from build123d import *

# Parameters (mm, degrees)
PAD_DEPTH = 27


with BuildPart() as part:
    # Sketch → Pad (new body)
    with BuildSketch(Plane.YZ):
        Polygon((0, 0), (0, 1), (3, 1), (3, 6), (5, 6), (5, 2), (7, 0), align=None)
    pad = extrude(amount=PAD_DEPTH)

    # Mirrored: Pad across Sketch V_Axis
    add(pad.mirror(Plane(origin=(0, 0, 0), x_dir=(1, 0, 0), z_dir=(0, 1, 0))))


solid = part.part
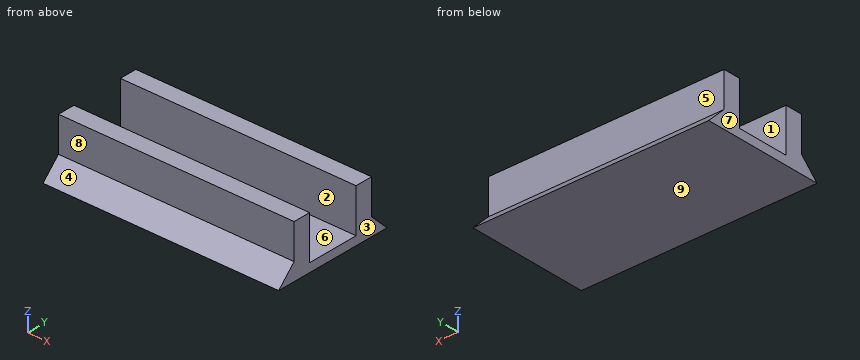
Input: part model. Units: mm. Frame: model coordinates. Face numbers are marked on the shaded views. A direction names the side the tool comes from. Give positions to 0.01 mm unless a question says otherwise; leave off trailing zeros. Loops run counter-clockwise (first coordinate to the right, second up) from the corner with the lowest first, then second, coordinate; pieces in that order, holes last. Notation, with made-up numbers: M 4.25,-33 L 16.25,-33 A10 ccw 16.25,-17 Z; hole C 1.25,61 d1. An arc over 180 degrees is marked long. Use one line per item in the form item = value.
1. Section query B-B, the plane x = 20.5. Return the cut outline in (y, z), and give its area (3 significant figures).
Numbers:
outline = M -7,0 L 7,0 L 5,2 L 5,6 L 3,6 L 3,1 L -3,1 L -3,6 L -5,6 L -5,2 Z
area = 34.0 mm²
2. Line query: L1, parallel to Y at x = 22.75, z = 3.4; L2, parallel to Z at x = 1.75, y = 1; L3, parallel to Y at x = 6.25, z = 1.4. Output: solid intervals per line, ascending.
Numbers:
L1 = -5 to -3, 3 to 5
L2 = 0 to 1
L3 = -5.6 to -3, 3 to 5.6
3. Reachability of the marked faces 5, 6, 7, 8 and 9 from +Z, -Z, +X, -X, +Y, -Y: full face, straight path, thin tool, end or side. Return the list, or none.
Numbers:
face_5 = +Z, +X, -X, +Y
face_6 = +Z, +X, -X
face_7 = +Z, -Z, -X, +Y, -Y
face_8 = +Z, +X, -X, -Y
face_9 = -Z, +X, -X, +Y, -Y
4. Pull-direction query (Y, two-part tool) for the marked faces 1, 2, 3 and 4; classes: released by +Y, released by -Y, zero draft, split by the parting line, or undercut.
Numbers:
face_1 = undercut
face_2 = undercut
face_3 = zero draft
face_4 = released by -Y
5. First-contact query: pin 1 (1 mm diameter, centred on y = -2, z = 2, fed in from -X); pin 2 (1.5 mm diameter, centred on x = 11, z = 4, fed in from +Y); pin 3 (8 mm diameter, centred on x = 15.5, y = 3, fed in from -Z); pin 4 (3 mm diameter, centred on x = 16, z = 4, fed in from -Y). Flat tips, straight axial feed; report the tip coordinate or a pass-through.
Numbers:
pin_1 = through
pin_2 = 5
pin_3 = 0
pin_4 = -5
6. Section query A-A, the plane z = 5.35. Return the cut outline in (x, y).
Numbers:
outline = M 0,-5 L 27,-5 L 27,-3 L 0,-3 Z; M 0,3 L 27,3 L 27,5 L 0,5 Z
7. Section query C-C, the plane y = 2.75. Return the cut outline in (x, z).
Numbers:
outline = M 0,0 L 27,0 L 27,1 L 0,1 Z
8. Section query D-D, the plane y = 5.25. Return the cut outline in (x, z).
Numbers:
outline = M 0,0 L 27,0 L 27,1.75 L 0,1.75 Z
